```python
from build123d import *

# Parameters (mm, degrees)
PAD008_DEPTH         = 15
SKETCH021_W          = 27.3
SKETCH021_H          = 27.3
POCKET006_DEPTH      = 12
POCKET007_DEPTH      = 5
SKETCH023_R          = 3.3665
POCKET008_DEPTH      = 68.001
SKETCH024_R          = 1.2
POCKET009_DEPTH      = 2.35
SKETCH026_R          = 1.2
POCKET010_DEPTH      = 33.951
POCKET010_DEPTH_BACK = 61.251
POCKET011_DEPTH      = 63.601
POCKET015_DEPTH      = 15.001
POCKET016_DEPTH      = 15.001


with BuildPart() as part:
    # Sketch020 → Pad008 (new body)
    with BuildSketch(Plane.XZ):
        with BuildLine():
            Line((-47.6, 1.5), (-47.6, 13.5))
            ThreePointArc((-46.1, 15), (-47.1606601718, 14.5606601718), (-47.6, 13.5))
            Line((-46.1, 15), (-23.5, 15))
            ThreePointArc((-23.5, 15), (-18.1966991411, 17.1966991411), (-16, 22.5))
            Line((-16, 22.5), (-16, 68))
            Line((-16, 68), (16, 68))
            Line((16, 68), (16, 22.5))
            ThreePointArc((16, 22.5), (18.1966991411, 17.1966991411), (23.5, 15))
            Line((23.5, 15), (46.1, 15))
            ThreePointArc((47.6, 13.5), (47.1606601718, 14.5606601718), (46.1, 15))
            Line((47.6, 13.5), (47.6, 1.5))
            ThreePointArc((46.1, 0), (47.1606601718, 0.4393398282), (47.6, 1.5))
            Line((46.1, 0), (17.5, 0))
            ThreePointArc((11.5, 6), (13.2573593129, 1.7573593129), (17.5, 0))
            Line((11.5, 9), (11.5, 6))
            ThreePointArc((11.5, 9), (9.7426406871, 13.2426406871), (5.5, 15))
            Line((-5.5, 15), (5.5, 15))
            ThreePointArc((-5.5, 15), (-9.7426406871, 13.2426406871), (-11.5, 9))
            Line((-11.5, 6), (-11.5, 9))
            ThreePointArc((-17.5, 0), (-13.2573593129, 1.7573593129), (-11.5, 6))
            Line((-17.5, 0), (-46.1, 0))
            ThreePointArc((-47.6, 1.5), (-47.1606601718, 0.4393398282), (-46.1, 0))
        make_face()
    extrude(amount=PAD008_DEPTH)

    # Sketch021 (on Face23 of Pad008) → Pocket006 (cut)
    with BuildSketch(Plane(origin=(0, 0, 0), x_dir=(1, 0, 0), z_dir=(0, 1, 0))):
        with Locations((0, -52)):
            Rectangle(SKETCH021_W, SKETCH021_H)
    extrude(amount=-POCKET006_DEPTH, mode=Mode.SUBTRACT)

    # Sketch022 (on Face29 of Pocket006) → Pocket007 (cut)
    with BuildSketch(Plane(origin=(0, -12, 0), x_dir=(1, 0, 0), z_dir=(0, 1, 0))):
        with BuildLine():
            ThreePointArc((-8, -56.0000000001), (-6.2100572838, -61.0433310949), (-1.6412028669, -63.8298437501))
            ThreePointArc((-1.6412028669, -63.8298437501), (0, -65.65), (1.6412028669, -63.8298437501))
            ThreePointArc((1.6412028669, -63.8298437501), (6.2100482063, -61.0433422724), (7.9999999999, -56.0000287985))
            Line((7.9999999999, -56.0000287985), (7.9999999999, -52.0000000001))
            ThreePointArc((8, -52.0000000001), (0, -44.0000000001), (-8, -52.0000000001))
            Line((-8, -52.0000000001), (-8, -56.0000000001))
        make_face()
    extrude(amount=-POCKET007_DEPTH, mode=Mode.SUBTRACT)

    # Sketch023 (on Face22 of Pocket007) → Pocket008 (cut, through all)
    with BuildSketch(Plane(origin=(0, 0, 0), x_dir=(1, 0, 0), z_dir=(0, 0, -1))):
        with Locations((38.1, 7.5)):
            Circle(SKETCH023_R)
        with Locations((-38.1, 7.5)):
            Circle(SKETCH023_R)
    extrude(amount=-POCKET008_DEPTH, mode=Mode.SUBTRACT)

    # Sketch024 (on Face13 of Pocket008) → Pocket009 (cut)
    with BuildSketch(Plane(origin=(0, 0, 68), x_dir=(-1, 0, 0), z_dir=(0, 0, 1))):
        with Locations((-6.15, 9.7)):
            Circle(SKETCH024_R)
        with Locations((6.15, 9.7)):
            Circle(SKETCH024_R)
    extrude(amount=-POCKET009_DEPTH, mode=Mode.SUBTRACT)

    # Sketch026 (on Face27 of Pocket009) → Pocket010 (cut, two sides)
    with BuildSketch(Plane(origin=(-13.65, 0, 0), x_dir=(0, 0, 1), z_dir=(1, 0, 0))) as pocket010_sk:
        with Locations((45.85, 9.7)):
            Circle(SKETCH026_R)
        with Locations((58.15, 9.7)):
            Circle(SKETCH026_R)
    extrude(amount=-POCKET010_DEPTH, mode=Mode.SUBTRACT)
    extrude(pocket010_sk.sketch, amount=POCKET010_DEPTH_BACK, mode=Mode.SUBTRACT)

    # Sketch027 (on Face15 of Pocket010) → Pocket011 (cut, through all)
    with BuildSketch(Plane(origin=(16, 0, 0), x_dir=(0, 0, 1), z_dir=(1, 0, 0))):
        with BuildLine():
            ThreePointArc((66.5, 6.5), (67.5606601718, 6.9393398282), (68, 8))
            Line((68, 8), (68, 0))
            Line((68, 0), (38.35, 0))
            ThreePointArc((38.35, 0), (39.1, 0.2009618943), (39.6490381057, 0.75))
            Line((42.5357894517, 5.75), (39.6490381057, 0.75))
            ThreePointArc((43.8348275573, 6.5), (43.0848275573, 6.2990381057), (42.5357894517, 5.75))
            Line((43.8348275573, 6.5), (66.5, 6.5))
        make_face()
    extrude(amount=-POCKET011_DEPTH, mode=Mode.SUBTRACT)

    # Sketch033 (on Face4 of Pocket011) → Pocket015 (cut, through all)
    with BuildSketch(Plane(origin=(0, 0, 0), x_dir=(1, 0, 0), z_dir=(0, 1, 0))):
        with BuildLine():
            ThreePointArc((19.9705882353, -15.8823529412), (24.185577345, -6.3911056638), (16, 0))
            Line((51, 0), (16, 0))
            Line((51, -22.5), (51, 0))
            Line((16, -22.5), (51, -22.5))
            ThreePointArc((19.9705882353, -15.8823529412), (17.0688030572, -18.6412818343), (16, -22.5))
        make_face()
    extrude(amount=-POCKET015_DEPTH, mode=Mode.SUBTRACT)

    # Sketch034 (on Face4 of Pocket015) → Pocket016 (cut, through all)
    with BuildSketch(Plane(origin=(0, 0, 0), x_dir=(1, 0, 0), z_dir=(0, 1, 0))):
        with BuildLine():
            ThreePointArc((-16, -1e-10), (-24.1855982279, -6.3910932116), (-19.9706006156, -15.8823463383))
            ThreePointArc((-16, -22.5), (-17.0688066666, -18.6412758186), (-19.9706006156, -15.8823463384))
            Line((-16, -22.5), (-51, -22.5))
            Line((-51, -22.5), (-51, -1e-10))
            Line((-51, -1e-10), (-16, -1e-10))
        make_face()
    extrude(amount=-POCKET016_DEPTH, mode=Mode.SUBTRACT)


solid = part.part
```
For this review, take the finished solid that the model builds, in its own axes (mm). A direction names the side the tool comes from. Coordinates: 2 decimals unless noted, no trailing zeros. Order: outer loops, then holes, each group sorted by start corner. A loop starts at its lowest first (then second) coordinate and runs counter-clockwise, first axis right, second up. Notation, with made-up numbers: (-14.5, 89.25) -> (-9.5, 89.25) arc R26 cw to (-9.5, 110.25) -> close; hole circle Ø9 at (25.25, 20.5). An arc over 180 degrees is marked (long way). Use CSV: the item, a comma, the result in double quotes. Start each with the question number.
Item 1: Wall thickness on probe 1 along X at (y, z) = (-9.7, 66.4); probe 2 along X at (y, z) = (-11.75, 41); probe 3 along Z at (x, y) = (-14.75, -9.7): over which ranges is each line inside the solid? List them lowest first.
Item 2: We need section A-A, the plane z = 61. Give the boundary of the cut face in (x, y) (3 decimals), then the cut area to 3 significant figures.
Item 3: Insertion check: pin 1 (3 mm diameter, centred on y = -9.7, z = 45.85, fed in from -X); pin 2 (11.5 mm diameter, centred on x = 6.5, z = 56, fed in from +Y); pin 3 (4 mm diameter, centred on x = 6.15, y = -9.7, fed in from -Z); pin 4 (3 mm diameter, centred on x = -6.15, y = -9.7, fed in from +Z). Each pin has a flat end and moves straight along its axis. Give the tip position at first contact, or say it passes through.
Item 4: For faces 4 (the face through (-13.062, -7.395, 1.962)), 5 (the face through (5.04, -9.24, 66.84)), 6 (the face through (-13.65, -9, 52)), 7 (the face through (0, -13, 44)), list the 3-axis set-ups (+Z, -Z, +X, -X, +Y, -Y) from which the entire face can be reached by the end or side of a thin tool; tool diameter is ignored.
Item 5: We need section B-B, the plane y = -9.7. Give the number of separate pieces and of enclosed holes in the cut face, then the cut area to 3 significant figures.
Item 6: We need section C-C, the plane z = 45.85. Give the boundary of the cut face in (x, y).
Item 7: Draft analysis for pull direction Y (two halves, no side actions). For faces 1 (the face through (-14.81, -9.24, 46.96)), 2 (the face through (-16, -9, 40)), 3 (the face through (0, 0, 19)), state which applies: pulls with the +Y half, pulls with the -Y half, needs draft (parallel to the pull), parting line crosses it, or undercut.
Derived:
1,probe 1,"x = -16 to -7.35, -4.95 to 4.95, 7.35 to 16"
1,probe 2,"x = -16 to -13.65, 13.65 to 16"
1,probe 3,"z = 0.67 to 44.65, 47.05 to 56.95, 59.35 to 68"
2,outline,"(-16, -15) -> (-6.245, -15) -> (-6.245, -12) -> (-13.65, -12) -> (-13.65, -6.5) -> (-16, -6.5) -> close; (6.245, -15) -> (16, -15) -> (16, -6.5) -> (13.65, -6.5) -> (13.65, -12) -> (6.245, -12) -> close"
2,area,"84.4 mm^2"
3,pin 1,"stops at x = -16"
3,pin 2,"stops at y = -12"
3,pin 3,"stops at z = 14.38"
3,pin 4,"stops at z = 68"
4,face 4,"-Z, +Y, -Y"
4,face 5,"+Z"
4,face 6,"+Y"
4,face 7,"+Y, -Y"
5,separate pieces,"6"
5,enclosed holes,"0"
5,area,"1,290 mm^2"
6,outline,"(-16, -15) -> (-5.12, -15) -> (-5.12, -12) -> (-13.65, -12) -> (-13.65, -10.9) -> (-16, -10.9) -> close; (-16, -8.5) -> (-13.65, -8.5) -> (-13.65, -6.5) -> (-16, -6.5) -> close; (5.12, -15) -> (16, -15) -> (16, -10.9) -> (13.65, -10.9) -> (13.65, -12) -> (5.12, -12) -> close; (13.65, -8.5) -> (16, -8.5) -> (16, -6.5) -> (13.65, -6.5) -> close"
7,face 1,"undercut"
7,face 2,"needs draft"
7,face 3,"pulls with the +Y half"
